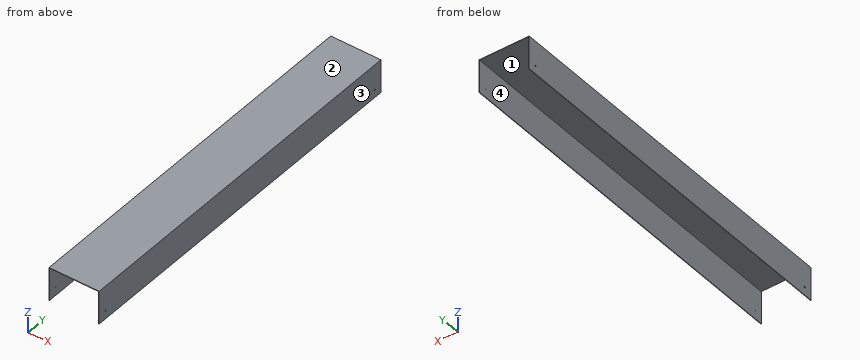
```python
from build123d import *

# Parameters (mm, degrees)
F1_DEPTH         = 1149.35
F3_D             = 4.7625
F3_DEPTH         = 25.4
F3_CSINK_D       = 9.525
F3_CSINK_ANGLE   = 90
F3_TIP           = 1.4307993491
F3_COPIES2_COUNT = 2


# Not quite as in the source:
# - a pattern or mirror of a feature is missing from the dataset's text; its kind, count and spacing are read off the source's solid


with BuildPart() as f1:
    # F0 (on Front) → F1 (new body, symmetric)
    with BuildSketch(Plane.XZ):
        Polygon((155.575, -103.1875), (155.575, 103.1875), (-155.575, 103.1875), (-155.575, -103.1875), (-152.4, -103.1875), (-152.4, 100.0125), (152.4, 100.0125), (152.4, -103.1875), align=None)
    extrude(amount=F1_DEPTH, both=True)

    # F3
    with Locations(Plane.YZ.offset(155.575)):
        with Locations((-1098.55, -52.3875)):
            f3 = CounterSinkHole(F3_D / 2, F3_CSINK_D / 2, depth=F3_DEPTH, counter_sink_angle=F3_CSINK_ANGLE)
            with Locations((0, 0, -(F3_DEPTH + F3_TIP / 2))):  # 118° drill point
                Cone(0, F3_D / 2, F3_TIP, mode=Mode.SUBTRACT)

    # F3_copies: F3 across plane
    add(f3.mirror(Plane(origin=(0, 0, 0), x_dir=(0, 0, -1), z_dir=(-1, 0, 0))), mode=Mode.SUBTRACT)

    # F3_copies1: F3 across plane
    add(f3.mirror(Plane.ZX), mode=Mode.SUBTRACT)

    # F3_copies2: F3 ×2 about axis
    f3_copies2_axis = Axis((0, 0, 0), (0, 0, 1))
    for i in range(1, F3_COPIES2_COUNT):
        add(f3.rotate(f3_copies2_axis, i * 360 / F3_COPIES2_COUNT), mode=Mode.SUBTRACT)


solid = f1.part
```
Design review of the part built by this model. Coordinates are the model's own, in mm. Face numbers are marked on the shaded views. Round coordinates to 2 decimals unless told otherwise and drop trailing zeros. Write each loop counter-clockwise with the first axis right and the second up, starting at its lowest first coordinate (ties: lowest second). Pieces come first, ordered by that corner, then holes. Notation, with made-up numbers: (68.5, 71) -> (89.5, 71) arc R19 cw to (89.5, 85) -> close; hole circle Ø9 at (29, -35.5). An arc over 180 degrees is marked (long way). Write item = value, one per line. Start each with the question number.
1) Mouldability with a two-part tool opening along X and no side actions: class the marked faces 1, 2, 3 and 4 as +X half, -X half, draft (parallel to the pull), parting line (faces both ways), or undercut.
2) Take a section at C-C, the plane x = 104. State the section outline as (y, z) points, plus the area to 3 significant figures.
3) Wall thickness on probe 1 along Z at (x, y) = (-152.9, 1098.55); probe 2 along X at (y, z) = (896, 92.5) (3 decimals); probe 3 along Z at (x, y) = (104.5, -624): over which ranges is each line inside the solid? List them lowest first. Write a range as from..to.
4) Clearance check with flat-ended pins moving along their axes: pin 1 (5.5 mm diameter, centred on y = -1098.55, z = -52.39, fed in from -X) (3 decimals); pin 2 (7.5 mm diameter, centred on y = 1098.55, z = -52.39, fed in from +X) (3 decimals); pin 3 (5.5 mm diameter, centred on y = 1098.55, z = -52.39, fed in from +X) (3 decimals). State where each tip first meets the part, or that it passes through.
5) Take a section at B-B, the plane y = 669.5. State the section outline as (x, z) points (1 decimal), plus the area to 3 significant figures.
6) Take a section at A-A, the plane z = 7.5. State the section outline as (x, y) points (3 decimals).
Results list:
q1.face_1 = undercut
q1.face_2 = draft
q1.face_3 = +X half
q1.face_4 = undercut
q2.outline = (-1149.35, 100.01) -> (1149.35, 100.01) -> (1149.35, 103.19) -> (-1149.35, 103.19) -> close
q2.area = 7,300 mm²
q3.probe_1 = -103.19..-54.77, -50.01..103.19
q3.probe_2 = -155.575..-152.4, 152.4..155.575
q3.probe_3 = 100.01..103.19
q4.pin_1 = -153.565
q4.pin_2 = 154.565
q4.pin_3 = 153.565
q5.outline = (-155.6, -103.2) -> (-152.4, -103.2) -> (-152.4, 100) -> (152.4, 100) -> (152.4, -103.2) -> (155.6, -103.2) -> (155.6, 103.2) -> (-155.6, 103.2) -> close
q5.area = 2,280 mm²
q6.outline = (-155.575, -1149.35) -> (-152.4, -1149.35) -> (-152.4, 1149.35) -> (-155.575, 1149.35) -> close; (152.4, -1149.35) -> (155.575, -1149.35) -> (155.575, 1149.35) -> (152.4, 1149.35) -> close
